Design review of the part built by this model. Coordinates are the model's own, in mm. A direction names the side the tool comes from. Coordinates: 2 decimals unless noted, no trailing zeros. Write each loop counter-clockwise with the first axis right and the second up, starting at its lowest first coordinate (ties: lowest second). Pieces come first, ordered by that corner, then holes. Notation, with made-up numbers: (12.5, 4.5) -> (63.5, 4.5) arc R34 cw to (63.5, 42.5) -> close; hole circle Ø3 at (36.25, 44). An arc over 180 degrees is marked (long way). Return JSON: item names as keys, results as strings. Group by question number.
from build123d import *

# Parameters (mm, degrees)
BOSS_EXTRUDE1_DEPTH        = 3
CUT_EXTRUDE1_DEPTH         = 10.5
M3_TAPPED_HOLE1_AT_2_COUNT = 2
M3_TAPPED_HOLE1_AT_2_PITCH = 6


with BuildPart() as part:
    # Sketch1 → Boss-Extrude1 (new body, symmetric)
    with BuildSketch(Plane(origin=(0, 0, 0), x_dir=(1, 0, 0), z_dir=(0, 1, 0))):
        with BuildLine():
            Line((0, -3.5), (0, 3.5))
            Line((0, 3.5), (14.8, 3.5))
            ThreePointArc((14.8, 3.5), (15.860660172, 3.939339828), (16.3, 5))
            Line((16.3, 5), (16.3, 6))
            Line((16.3, 6), (23.5, 6))
            Line((23.5, 6), (23.5, -6))
            Line((23.5, -6), (16.3, -6))
            Line((16.3, -6), (16.3, -5))
            ThreePointArc((16.3, -5), (15.860660172, -3.939339828), (14.8, -3.5))
            Line((14.8, -3.5), (0, -3.5))
        make_face()
    extrude(amount=BOSS_EXTRUDE1_DEPTH, both=True)

    # Sketch2 → Cut-Extrude1 (cut, through all)
    with BuildSketch(Plane.XY.offset(3.5)):
        with BuildLine():
            ThreePointArc((7.847845894, 1.375), (7.45, 0), (7.847845894, -1.375))
            Line((7.847845894, -1.375), (10.025, -1.375))
            Line((10.025, -1.375), (10.025, 1.375))
            Line((10.025, 1.375), (7.847845894, 1.375))
        make_face()
        with BuildLine():
            Line((10.025, -1.375), (7.847845894, -1.375))
            ThreePointArc((7.847845894, -1.375), (10.740700069, -2.473539652), (12.6, 0))
            ThreePointArc((12.6, 0), (10.740700069, 2.473539652), (7.847845894, 1.375))
            Line((7.847845894, 1.375), (10.025, 1.375))
            Line((10.025, 1.375), (10.025, -1.375))
        make_face()
        with BuildLine():
            Line((0, 1.375), (0, -1.375))
            Line((0, -1.375), (7.847845894, -1.375))
            ThreePointArc((7.847845894, -1.375), (7.45, 0), (7.847845894, 1.375))
            Line((7.847845894, 1.375), (0, 1.375))
        make_face()
    extrude(amount=-CUT_EXTRUDE1_DEPTH, mode=Mode.SUBTRACT)

    # Sketch5 → M3 Tapped Hole1 (revolve, cut)
    with BuildSketch(Plane(origin=(20, 3, -3), x_dir=(0, 0, 1), z_dir=(1, 0, 0))):
        Polygon((0, 0), (0, 6), (1.75, 6), (1.25, 5.5), (1.25, 0.5), (1.75, 0), align=None)
    m3_tapped_hole1 = revolve(axis=Axis((20, 9.35, -3), (0, -1, 0)), mode=Mode.SUBTRACT)

    # M3 Tapped Hole1 at 2: M3 Tapped Hole1 ×2
    with Locations(*[(0, 0, i * M3_TAPPED_HOLE1_AT_2_PITCH) for i in range(1, M3_TAPPED_HOLE1_AT_2_COUNT)]):
        add(m3_tapped_hole1, mode=Mode.SUBTRACT)

    # Mirror1: part across plane


with BuildPart() as part_1:
    add(part.part)
    add(part.part.mirror(Plane(origin=(0, 0, 0), x_dir=(0, 0, 1), z_dir=(1, 0, 0))))


solid = part_1.part
Q1. For P1, Ø3, axis at x = -20, z = 3, coming from the +Y side; P2, Ø4, axis at x = 20, z = 3, coming from the -Y side, all flat-tipped, find the tip position at first contact; note any pin that passes through.
Q2. For faces 4 (the cylindrical face through (15.85, 0.04, -3.93)), 5 (the flat face through (0, 2, 3.5)), 6 (the flat face through (0, 1.375, 0)), list the 3-axis set-ups (+Z, -Z, +X, -X, +Y, -Y) from which the entire face can be reached by the end or side of a thin tool; tool diameter is ignored.
Q3. We need section D-D on x = -20. Write out the cut boundary in (y, z).
Q4. We need section A-A on x = 3. Write out the cut boundary in (y, z) (3 decimals), plus the area to 4 significant figures.
Q5. Wall thickness on L1, parallel to X at y = -0.1, z = 3; L2, parallel to Z at x = 20, y = -1.25; L3, parallel to X at y = 0.1, z = 1.5: over which ranges is each line inside the solid? List them lowest first.
Q6. We need section B-B on z = -3. Write out the cut boundary in (x, y) (3 decimals), plus the area to 3 significant figures.
Q7. We need section C-C on y = 0.7. Write out the cut boundary in (x, z).
Q8. The part is to be moulded in two halves that separate along X. For faces 1 (the flat face through (-23.5, 0, 0)), 2 (the flat face through (20, 0, -6)), 3 (the flat face through (16.3, 0, -5.5)), say which applies: +X half, -X half, draft (parallel to the pull), parting line (faces both ways), or undercut.
Findings below:
{
 "1": {"P1": "stops at y = 2.75", "P2": "stops at y = -3"},
 "2": {"face 4": "-Z, +Y, -Y", "face 5": "+Z, +Y, -Y", "face 6": "+Z, -Z"},
 "3": {"outline": "(-3, -6) -> (3, -6) -> (3, -4.75) -> (2.5, -4.25) -> (-2.5, -4.25) -> (-3, -4.75) -> close; (-3, -1.25) -> (-2.5, -1.75) -> (2.5, -1.75) -> (3, -1.25) -> (3, 1.25) -> (2.5, 1.75) -> (-2.5, 1.75) -> (-3, 1.25) -> close; (-3, 4.75) -> (-2.5, 4.25) -> (2.5, 4.25) -> (3, 4.75) -> (3, 6) -> (-3, 6) -> close"},
 "4": {"outline": "(-3, -3.5) -> (-1.375, -3.5) -> (-1.375, 3.5) -> (-3, 3.5) -> close; (1.375, -3.5) -> (3, -3.5) -> (3, 3.5) -> (1.375, 3.5) -> close", "area": "22.75 mm^2"},
 "5": {"L1": "x = -23.5 to -21.25, -18.75 to -12.6, 12.6 to 18.75, 21.25 to 23.5", "L2": "z = -6 to -4.25, -1.75 to 1.75, 4.25 to 6", "L3": "x = -23.5 to -12.6, 12.6 to 23.5"},
 "6": {"outline": "(-23.5, -3) -> (-21.75, -3) -> (-21.25, -2.5) -> (-21.25, 2.5) -> (-21.75, 3) -> (-23.5, 3) -> close; (-18.75, -2.5) -> (-18.25, -3) -> (18.25, -3) -> (18.75, -2.5) -> (18.75, 2.5) -> (18.25, 3) -> (-18.25, 3) -> (-18.75, 2.5) -> close; (21.25, -2.5) -> (21.75, -3) -> (23.5, -3) -> (23.5, 3) -> (21.75, 3) -> (21.25, 2.5) -> close; hole (-7.848, -1.375) -> (7.848, -1.375) arc R2.575 ccw (long way) to (7.848, 1.375) -> (-7.848, 1.375) arc R2.575 ccw (long way) to start", "area": "168 mm^2"},
 "7": {"outline": "(-23.5, -6) -> (-16.3, -6) -> (-16.3, -5) arc R1.5 cw to (-14.8, -3.5) -> (-12.5, -3.5) -> (-12.5, 3.5) -> (-14.8, 3.5) arc R1.5 cw to (-16.3, 5) -> (-16.3, 6) -> (-23.5, 6) -> close; (12.5, -3.5) -> (14.8, -3.5) arc R1.5 cw to (16.3, -5) -> (16.3, -6) -> (23.5, -6) -> (23.5, 6) -> (16.3, 6) -> (16.3, 5) arc R1.5 cw to (14.8, 3.5) -> (12.5, 3.5) -> close; hole circle Ø2.5 at (-20, -3); hole circle Ø2.5 at (-20, 3); hole circle Ø2.5 at (20, -3); hole circle Ø2.5 at (20, 3)"},
 "8": {"face 1": "-X half", "face 2": "draft", "face 3": "undercut"}
}
